from build123d import *

# Parameters (mm, degrees)
F0_W     = 76.2
F0_H     = 76.2
F0_W_2   = 70.104
F0_H_2   = 70.104
F1_DEPTH = 241.3
F3_DEPTH = 76.201
F4_W     = 165.1
F4_H     = 76.2
F5_DEPTH = 76.201
F6_R     = 3.175


with BuildPart() as f1:
    # F0 (on Front) → F1 (new body)
    with BuildSketch(Plane.XZ):
        Rectangle(F0_W, F0_H)
        Rectangle(F0_W_2, F0_H_2, mode=Mode.SUBTRACT)
    extrude(amount=F1_DEPTH)

    # F2 (on face) → F3 (cut, through all)
    with BuildSketch(Plane.YZ.offset(38.1)):
        Polygon((0, -38.1), (0, 38.1), (-57.15, -38.1), align=None)
    extrude(amount=-F3_DEPTH, mode=Mode.SUBTRACT)

    # F4 (on face) → F5 (cut, through all)
    with BuildSketch(Plane.YZ.offset(38.1)):
        with Locations((-158.75, 0)):
            Rectangle(F4_W, F4_H)
    extrude(amount=-F5_DEPTH, mode=Mode.SUBTRACT)

    # F6
    f6_edges = [f1.edges().sort_by_distance(p)[0] for p in [
        (38.1, -38.1, 38.1),
        (-38.1, -38.1, 38.1),
        (-38.1, -66.675, -38.1),
        (38.1, -66.675, -38.1),
    ]]
    fillet(f6_edges, radius=F6_R)


solid = f1.part
Can you work these out from the model? Positions are in its coordinate system, mm. A direction names the side the tool comes from. Coordinates: 2 decimals unless noted, no trailing zeros. Loops run counter-clockwise (first coordinate to the right, second up) from the corner with the lowest first, then second, coordinate; pieces in that order, holes last. Notation, with made-up numbers: M -10,81 L 9,81 A22 ccw 9,90 Z; hole C 27,12.25 d4. An arc over 180 degrees is marked long. Answer as CSV lines item,"result". Start each with the question number.
1. Suppose I cut it at D-D, the plane y = -27. List the corners of the cut face in (x, z) for me (3 decimals).
2. Thinking about a two-plate mould opening in X: for faces 1 (the face through (35.052, -47, 7)), 2 (the face through (-38.1, -47, 7)), 3 (the face through (37.15, -65.63, -37.19)), 4 (the face through (0, -39, 35.052)), which applies, +X half, -X half, draft (parallel to the pull), parting line (faces both ways), or undercut?
3. For faces 5 (the face through (38.1, -47, 7)), 6 (the face through (0, -65, -35.052)), which set-ups out of +Z, -Z, +X, -X, +Y, -Y let a thin tool reach every point of the face, with its end or its side?
4. For pin 1 Ø5 at (x, y) = (2.5, -11) entering from -Z, with a flat end and sliding along its axis, tell me the tip position at first contact or that it passes through.
5. Suppose I cut it at B-B, the plane z = 22. List the corners of the cut face in (x, y) for me (3 decimals).
6. If I drill on probe 1 along X at (y, z) = (-50.5, -26); probe 2 along Z at (x, y) = (22, -48), over which ranges is the centre line in solid material (lowest first)? Write a range as [from, to].
7. Suppose I cut it at C-C, the plane y = -67. List the corners of the cut face in (x, z) for me (3 decimals), plus the area to 3 significant figures.
8. Suppose I cut it at A-A, the plane x = 2.5. List the corners of the cut face in (y, z) for me.
Output:
1,outline,"M -38.1,2.1 L -35.052,2.1 L -35.052,35.052 L 35.052,35.052 L 35.052,2.1 L 38.1,2.1 L 38.1,34.925 A3.175 ccw 34.925,38.1 L -34.925,38.1 A3.175 ccw -38.1,34.925 Z"
2,face 1,"undercut"
2,face 2,"-X half"
2,face 3,"+X half"
2,face 4,"undercut"
3,face 5,"+Z, -Z, +X, +Y, -Y"
3,face 6,"+Y, -Y"
4,pin 1,"stops at z = 35.05"
5,outline,"M -38.1,-76.2 L -35.052,-76.2 L -35.052,-12.075 L -38.1,-12.075 Z; M 35.052,-76.2 L 38.1,-76.2 L 38.1,-12.075 L 35.052,-12.075 Z"
6,probe 1,"x = [-38.1, -35.05], [35.05, 38.1]"
6,probe 2,"z = [35.05, 38.1]"
7,outline,"M -38.1,-34.925 A3.175 ccw -34.925,-38.1 L 34.925,-38.1 A3.175 ccw 38.1,-34.925 L 38.1,34.925 A3.175 ccw 34.925,38.1 L -34.925,38.1 A3.175 ccw -38.1,34.925 Z; hole M -35.052,-35.052 L 35.052,-35.052 L 35.052,35.052 L -35.052,35.052 Z"
7,area,"883 mm^2"
8,outline,"M -76.2,-38.1 L -57.15,-38.1 L -54.86,-35.05 L -76.2,-35.05 Z; M -76.2,35.05 L -2.29,35.05 L 0,38.1 L -76.2,38.1 Z"
